from build123d import *

# Parameters (mm, degrees)
F1_R     = 1
F1_R_2   = 4
F2_DEPTH = 4


# Not quite as in the source:
# - a feature names something its author has since deleted; it is built from what else it names


with BuildPart() as f2:
    # F1 (on Front) → F2 (new body)
    with BuildSketch(Plane.XZ):
        with BuildLine():
            ThreePointArc((54.0977004839, -4.1335701552), (56.766858502, 3.238282099), (49.9672364551, 7.1413258089))
            Line((49.9672364551, 7.1413258089), (9.0970295176, 4.3491148777))
            Line((9.0970295176, 4.3491148777), (-50.8374237274, -3.466212469))
            ThreePointArc((-50.8374237274, -3.466212469), (-52.8544943464, -4.3378942821), (-54.1067810637, -6.1434914253))
            Line((-54.1067810637, -6.1434914253), (-62.5583549212, -30.968136056))
            ThreePointArc((-62.5583549212, -30.968136056), (-63.2874110026, -31.9497789492), (-64.4516400514, -32.3235653341))
            Line((-64.4516400514, -32.3235653341), (-66.6727852076, -32.3235653341))
            ThreePointArc((-66.6727852076, -32.3235653341), (-67.1968351707, -32.5406339362), (-67.4139037728, -33.0646838993))
            Line((-67.4139037728, -33.0646838993), (-67.4139037728, -36.8838813156))
            ThreePointArc((-67.4139037728, -36.8838813156), (-67.1968351707, -37.4079312787), (-66.6727852076, -37.6249998808))
            Line((-66.6727852076, -37.6249998808), (-62.3935461021, -37.6249998808))
            ThreePointArc((-62.3935461021, -37.6249998808), (-62.0598715448, -37.6530309942), (-61.7355502568, -37.736338591))
            Line((-61.7355502568, -37.736338591), (-37.2162681051, -46.2786780104))
            ThreePointArc((-37.2162681051, -46.2786780104), (-36.8173856222, -46.3731607561), (-36.4076181612, -46.3843344843))
            Line((-36.4076181612, -46.3843344843), (-13.7597462162, -44.6734763682))
            Line((-13.7597462162, -44.6734763682), (5.0197247755, -42.1101055891))
            ThreePointArc((5.0197247755, -42.1101055891), (5.6431122997, -41.9176107253), (6.1713765615, -41.5347228206))
            Line((6.1713765615, -41.5347228206), (8.2269536442, -39.4559054448))
            ThreePointArc((8.2269536442, -39.4559054448), (8.625280402, -38.9562994549), (8.9087680688, -38.3836694749))
            Line((8.9087680688, -38.3836694749), (16.3488967626, -18.1892685938))
            ThreePointArc((16.3488967626, -18.1892685938), (17.208766797, -16.9510123668), (18.5623472371, -16.2873294968))
            Line((18.5623472371, -16.2873294968), (40.5820753294, -11.7802791422))
            ThreePointArc((40.5820753294, -11.7802791422), (41.0467937044, -11.6453208131), (41.4837674916, -11.4374005686))
            Line((41.4837674916, -11.4374005686), (54.0977004839, -4.1335701552))
        make_face()
        with Locations((-64.3514022231, -34.8506011069)):
            Circle(F1_R, mode=Mode.SUBTRACT)
        with BuildLine():
            ThreePointArc((-16.7472230261, -4.91411715), (-15.1379574632, -5.4133219884), (-14.4811960302, -6.9649680637))
            Line((-14.4811960302, -6.9649680637), (-14.5219445245, -8.1491333606))
            ThreePointArc((-14.5219445245, -8.1491333606), (-14.32171034, -8.5009617779), (-13.9174035461, -8.4806398607))
            Line((-13.9174035461, -8.4806398607), (-8.2003281839, -4.5523469385))
            ThreePointArc((-8.2003281839, -4.5523469385), (-6.3639342341, -3.6131535453), (-4.348447762, -3.1747002983))
            Line((-4.348447762, -3.1747002983), (-1.8018096929, -2.9578907207))
            ThreePointArc((-1.8018096929, -2.9578907207), (-0.3607692656, -3.4067953543), (0.3561826933, -4.7349868962))
            Line((0.3561826933, -4.7349868962), (0.5668963829, -6.67740348))
            Line((0.5668963829, -6.67740348), (0.672921323, -6.6315499412))
            ThreePointArc((0.672921323, -6.6315499412), (1.9999899765, -6.5396114649), (3.091186979, -7.3004353579))
            Line((3.091186979, -7.3004353579), (9.1316822834, -15.7097849605))
            ThreePointArc((9.1316822834, -15.7097849605), (9.4794348377, -16.5438272503), (9.4245987558, -17.4457980836))
            ThreePointArc((9.4245987558, -17.4457980836), (9.3536544385, -17.6453573177), (9.2620047676, -17.8362953231))
            Line((9.2620047676, -17.8362953231), (4.5568440785, -29.1365425288))
            Line((4.5568440785, -29.1365425288), (3.6719114619, -31.2618593858))
            ThreePointArc((3.6719114619, -31.2618593858), (3.5914700409, -31.4944450482), (3.483071784, -31.715390133))
            Line((3.483071784, -31.715390133), (1.6890171815, -36.0241187498))
            ThreePointArc((1.6890171815, -36.0241187498), (1.0710114326, -36.8336930562), (0.1344541234, -37.2339455637))
            Line((0.1344541234, -37.2339455637), (-11.7459257638, -38.985923444))
            Line((-11.7459257638, -38.985923444), (-39.1007720975, -41.6174277811))
            ThreePointArc((-39.1007720975, -41.6174277811), (-39.5919940555, -41.6040344694), (-40.0651227377, -41.4712653355))
            Line((-40.0651227377, -41.4712653355), (-48.4746967713, -37.9479731273))
            ThreePointArc((-48.4746967713, -37.9479731273), (-48.9998078369, -37.6249470931), (-49.401585452, -37.1573337934))
            Line((-49.401585452, -37.1573337934), (-55.2931292161, -27.6564465473))
            ThreePointArc((-55.2931292161, -27.6564465473), (-55.5850730561, -26.7847906202), (-55.4562690933, -25.874612176))
            Line((-55.4562690933, -25.874612176), (-48.8776308187, -9.0366472667))
            ThreePointArc((-48.8776308187, -9.0366472667), (-48.2268856759, -8.1736364118), (-47.2221234757, -7.7752523038))
            Line((-47.2221234757, -7.7752523038), (-19.7747927159, -4.91411715))
            Line((-19.7747927159, -4.91411715), (-16.7472230261, -4.91411715))
        make_face(mode=Mode.SUBTRACT)
        with BuildLine():
            ThreePointArc((7.2113401452, -7.3855209262), (6.7341998146, -4.9209260348), (8.2972601063, -2.9565601324))
            Line((8.2972601063, -2.9565601324), (10.5244084197, -1.8336281786))
            ThreePointArc((10.5244084197, -1.8336281786), (11.0639592867, -1.6241164689), (11.6337015289, -1.5221161154))
            Line((11.6337015289, -1.5221161154), (42.2805400914, 0.9513819838))
            ThreePointArc((42.2805400914, 0.9513819838), (44.1319918409, 0.4924203394), (45.3325095049, -0.989901053))
            ThreePointArc((45.3325095049, -0.989901053), (45.4924194241, -1.3771741585), (45.6785557512, -1.752547184))
            ThreePointArc((45.6785557512, -1.752547184), (45.9010642846, -4.0736832448), (44.3940516522, -5.8530358197))
            Line((44.3940516522, -5.8530358197), (12.9439963939, -12.3211824174))
            ThreePointArc((12.9439963939, -12.3211824174), (11.2477431433, -12.1769167526), (9.9030954921, -11.132881137))
            Line((9.9030954921, -11.132881137), (7.2113401452, -7.3855209262))
        make_face(mode=Mode.SUBTRACT)
        with Locations((51.0432839383, 1.1414983302)):
            Circle(F1_R_2, mode=Mode.SUBTRACT)
    extrude(amount=F2_DEPTH)


solid = f2.part
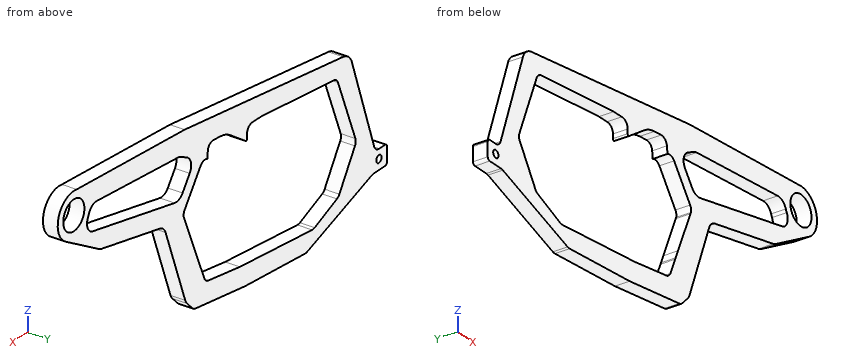
Could you check a few things on this model? Use its own coordinates, in mm. Give positions to 0.01 mm unless a question says otherwise; leave off trailing zeros. Write each loop counter-clockwise with the first axis right and the second up, starting at its lowest first coordinate (ties: lowest second). Pieces come first, ordered by that corner, then holes. Notation, with made-up numbers: (3.25, 49.25) -> (53.25, 49.25) arc R14 ccw to (53.25, 59.25) -> close; hole circle Ø11 at (-1, 3). An arc over 180 degrees is marked (long way). Write each question's results on one line, items separated by ' | '. Start each with the question number.
Q1. I'm going to push flat-ended pins straight in: pin 1 Ø0.7 at (x, y) = (-65.5, -3) entering from +Z; pin 2 Ø1.5 at (y, z) = (-0.5, -10.5) entering from +X; pin 3 Ø1.2 at (x, y) = (-64, -3) entering from -Z (3 decimals). Where does each tip first touch, or does it pass through?
Q2. Suppose I cut it at A-A, the plane x = 28. List the corners of the cut face in (y, z) for me.
Q3. I need wall thicknesses on probe 1 along X at (y, z) = (-1.35, -4.5); probe 2 along X at (y, z) = (-3.1, -36.5); probe 3 along X at (y, z) = (-2.05, -33.5). Which ranges of each line are inside material? Lowest first, please.
Q4. Suppose I cut it at B-B, the plane z = -24. List the corners of the cut face in (x, y) for me.
Q5. Suppose I cut it at C-C, the plane y = -2.6. State how many separate pieces and enclosed holes the cut face has, and give its area (3 significant figures).
Outcome:
1) pin 1: z = -32.32 | pin 2: x = 44.4 | pin 3: z = -37.625
2) outline: (-4, -14.36) -> (0, -14.36) -> (0, -9.22) -> (-4, -9.22) -> close; (-4, -0.2) -> (0, -0.2) -> (0, 5.64) -> (-4, 5.64) -> close
3) probe 1: -53.04 to -8.12, 0.32 to 6.87, 45.73 to 53.46 | probe 2: -67.41 to -49.81, 1.41 to 9.6 | probe 3: -67.41 to -51.67, 2.74 to 10.71
4) outline: (-60.19, -4) -> (-54.72, -4) -> (-54.72, 0) -> (-60.19, 0) -> close; (6.7, -4) -> (14.21, -4) -> (14.21, 0) -> (6.7, 0) -> close
5) separate pieces: 1 | enclosed holes: 4 | area: 1,610 mm2
